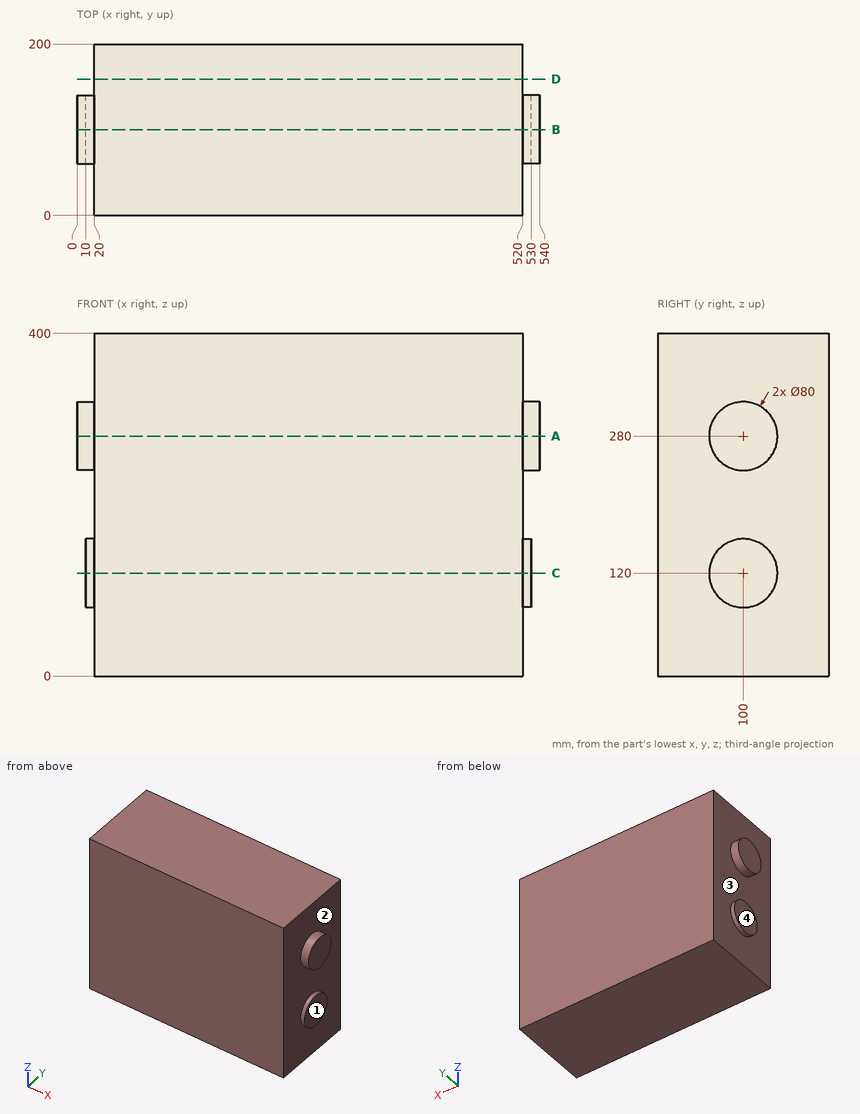
Drawing for the job (mm, zero at the part's lowest x, y, z). A direction names the side the tool comes from. Round coordinates to 2 decimals unless told otherwise and drop trailing zeros. Write each loop counter-clockwise with the first axis right and the second up, starting at its lowest first coordinate (ties: lowest second). Pieces come first, ordered by that corner, then holes. Notation, with made-up numbers: M -15.5,-36 L 20.5,-36 A19 cw 20.5,1 Z; hole C 58,-12.5 d8. An arc over 180 degrees is marked long. Put each result on its own line as item: value.
Item 1: Cut at D-D (y = 159). List the corners of the cut face in (x, z).
Responses:
outline: M 20,0 L 520,0 L 520,400 L 20,400 Z
Item 2: Tool access for the marked faces 1, 2, 3 and 4: list every direction of +Z, -Z, +X, -X, +Y, -Y with a clear straight run to the whole face (end or side of a thin tool).
Responses:
face 1: -Z, +X, +Y, -Y
face 2: +X
face 3: -X
face 4: -Z, -X, +Y, -Y
Item 3: Flat gauge pins, fed straight in: P1, Ø6, axis at y = 42.5, z = 173, coming from the -X side; P2, Ø5, axis at y = 141.5, z = 228, coming from the +X side; P3, Ø1, axis at x = 175.5, z = 214.5, coming from the -Y side; P4, Ø1, axis at y = 112.5, z = 93.5, coming from the -X side. Where does each tip first touch, or does it go through?
Responses:
P1: x = 20
P2: x = 520
P3: y = 0
P4: x = 10
Item 4: Probe L1, parallel to X at y = 175, z = 356; L2, parallel to X at y = 93, z = 90.5. List the from-to ranges inside material, lowest first. Write a range as from..to.
Responses:
L1: 20..520
L2: 10..530
Item 5: Cut at B-B (y = 100). List the corners of the cut face in (x, z).
Responses:
outline: M 0,240 L 20,240 L 20,160 L 10,160 L 10,80 L 20,80 L 20,0 L 520,0 L 520,80 L 530,80 L 530,160 L 520,160 L 520,240 L 540,240 L 540,320 L 520,320 L 520,400 L 20,400 L 20,320 L 0,320 Z
Item 6: Cut at A-A (z = 280). List the corners of the cut face in (x, y).
Responses:
outline: M 0,60 L 20,60 L 20,0 L 520,0 L 520,60 L 540,60 L 540,140 L 520,140 L 520,200 L 20,200 L 20,140 L 0,140 Z
Item 7: Cut at C-C (z = 120). List the corners of the cut face in (x, y).
Responses:
outline: M 10,60 L 20,60 L 20,0 L 520,0 L 520,60 L 530,60 L 530,140 L 520,140 L 520,200 L 20,200 L 20,140 L 10,140 Z
